Here's how the part is built. I have some questions about the finished solid (model axes, mm). Face numbers are marked on the shaded views. Give positions to 0.01 mm unless a question says otherwise; leave off trailing zeros. Order: outer loops, then holes, each group sorted by start corner. A loop starts at its lowest first (then second) coordinate and runs counter-clockwise, first axis right, second up. Notation, with made-up numbers: (35.25, -37.5) -> (55.25, -37.5) arc R15 ccw to (55.25, -17.5) -> close; hole circle Ø4 at (80.5, -14). An arc over 180 degrees is marked (long way). Write each question's results on one line, items separated by ' | '. Start each with the question number.
Q1. I'm going to push flat-ended pins straight in: pin 1 (1 mm diameter, centred on x = -1, y = 1, fed in from +Z); pin 2 (1 mm diameter, centred on x = -2.5, y = 4, fed in from -Z); pin 3 (2.5 mm diameter, centred on x = -10, z = 0, fed in from -Y). Where does each tip first touch, or does it pass through?
Q2. Imagine slicing it at C-C, the plane y = 0.85. Please give me the cut outline in (x, z), then the cut area to 3 significant figures.
Q3. Thinking about a two-plate mould opening in X: for the marked faces 1, 2 and 3, which applies, pulls with the +X half, pulls with the -X half, needs draft (parallel to the pull), parting line crosses it, or undercut?
Q4. Imagine slicing it at B-B, the plane x = 0. Please give me the cut outline in (y, z), then the cut area to 3 significant figures.
Q5. Imagine slicing it at A-A, the plane z = 0. Please give me the cut outline in (x, y).
Q6. I need wall thicknesses on line 1 along Y through (x, z) = (7, 9); line 2 along Z through (x, y) = (2, 4.95); line 3 along Z through (x, y) = (0.5, 2.5). Which ranges of each line are inside material? Lowest first, please. Write a range as [from, to].
```python
from build123d import *

# Parameters (mm, degrees)
SKETCH1_R           = 7.5
SKETCH1_R_2         = 5.5
BOSS_EXTRUDE1_DEPTH = 4
SKETCH2_R           = 13
SKETCH2_R_2         = 5.5
BOSS_EXTRUDE2_DEPTH = 1.4
SKETCH3_R           = 1.09
CUT_EXTRUDE1_DEPTH  = 20.161419572
CIRPATTERN1_COUNT   = 4
FILLET1_R           = 0.25


with BuildPart() as part:
    # Sketch1 → Boss-Extrude1 (new body)
    with BuildSketch(Plane(origin=(0, 0, 0), x_dir=(1, 0, 0), z_dir=(0, 1, 0))):
        with Locations(Location((0, 0, 0), (0, 0, 270))):
            Circle(SKETCH1_R)
        with Locations(Location((0, 0, 0), (0, 0, 270))):
            Circle(SKETCH1_R_2, mode=Mode.SUBTRACT)
    extrude(amount=BOSS_EXTRUDE1_DEPTH)

    # Sketch2 → Boss-Extrude2 (add)
    with BuildSketch(Plane(origin=(0, 4, 0), x_dir=(1, 0, 0), z_dir=(0, 1, 0))):
        with Locations(Location((0, 0, 0), (0, 0, 270))):
            Circle(SKETCH2_R)
        with Locations(Location((0, 0, 0), (0, 0, 270))):
            Circle(SKETCH2_R_2, mode=Mode.SUBTRACT)
    extrude(amount=BOSS_EXTRUDE2_DEPTH)

    # Sketch3 → Cut-Extrude1 (cut, through all)
    with BuildSketch(Plane(origin=(0, 5.4, 0), x_dir=(1, 0, 0), z_dir=(0, 1, 0))):
        with Locations(Location((0, 10, 0), (0, 0, 270))):
            Circle(SKETCH3_R)
    cut_extrude1 = extrude(amount=-CUT_EXTRUDE1_DEPTH, mode=Mode.SUBTRACT)

    # CirPattern1: Cut-Extrude1 ×4 about axis
    cirpattern1_axis = Axis((0, 0, 0), (0, 1, 0))
    for i in range(1, CIRPATTERN1_COUNT):
        add(cut_extrude1.rotate(cirpattern1_axis, i * 360 / CIRPATTERN1_COUNT), mode=Mode.SUBTRACT)

    # Fillet1
    fillet1_edges = [part.edges().sort_by_distance(p)[0] for p in [
        (0, 4, -13),
        (0, 5.4, -13),
    ]]
    fillet(fillet1_edges, radius=FILLET1_R)


solid = part.part
```
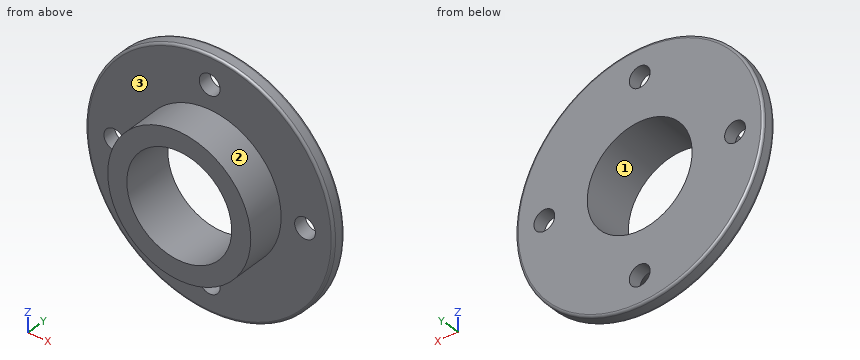
Geometry check:
1) pin 1: z = 7.48 | pin 2: z = -12.84 | pin 3: y = 4
2) outline: circle Ø15 at (0, 0); hole circle Ø11 at (0, 0) | area: 81.7 mm²
3) face 1: undercut | face 2: parting line crosses it | face 3: needs draft
4) outline: (0, -7.5) -> (4, -7.5) -> (4, -8.91) -> (5.4, -8.91) -> (5.4, -5.5) -> (0, -5.5) -> close; (0, 5.5) -> (5.4, 5.5) -> (5.4, 8.91) -> (4, 8.91) -> (4, 7.5) -> (0, 7.5) -> close; (4, -12.75) arc R0.25 ccw to (4.25, -13) -> (5.15, -13) arc R0.25 ccw to (5.4, -12.75) -> (5.4, -11.09) -> (4, -11.09) -> close; (4, 11.09) -> (5.4, 11.09) -> (5.4, 12.75) arc R0.25 ccw to (5.15, 13) -> (4.25, 13) arc R0.25 ccw to (4, 12.75) -> close | area: 30.8 mm²
5) outline: (-13, 4.25) arc R0.25 ccw to (-12.75, 4) -> (-11.09, 4) -> (-11.09, 5.4) -> (-12.75, 5.4) arc R0.25 ccw to (-13, 5.15) -> close; (-8.91, 4) -> (-7.5, 4) -> (-7.5, 0) -> (-5.5, 0) -> (-5.5, 5.4) -> (-8.91, 5.4) -> close; (5.5, 0) -> (7.5, 0) -> (7.5, 4) -> (8.91, 4) -> (8.91, 5.4) -> (5.5, 5.4) -> close; (11.09, 4) -> (12.75, 4) arc R0.25 ccw to (13, 4.25) -> (13, 5.15) arc R0.25 ccw to (12.75, 5.4) -> (11.09, 5.4) -> close
6) line 1: [4, 5.4] | line 2: [-12.85, -5.12], [5.12, 12.85] | line 3: [-7.48, -5.48], [5.48, 7.48]
